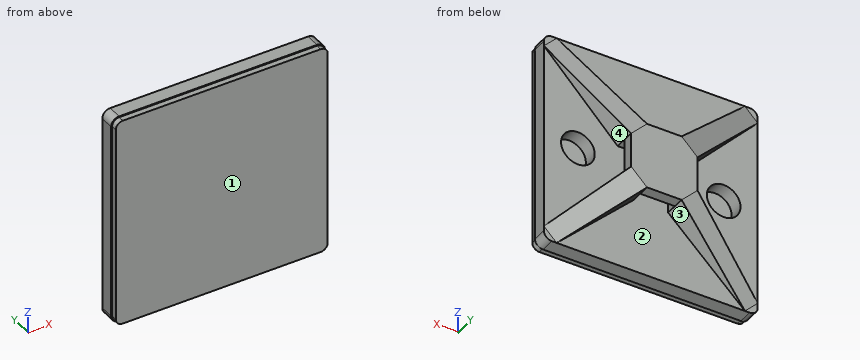
from build123d import *

# Parameters (mm, degrees)
BOSS_EXTRUDE1_DEPTH   = 1.905
BOSS_EXTRUDE2_DEPTH   = 2.921
CUT_EXTRUDE2_DEPTH    = 21.205576272
CIRPATTERN3_COUNT     = 4
SKETCH5_W             = 4.62591911
SKETCH5_H             = 1.4605
CUT_EXTRUDE3_DEPTH    = 19.7198
CIRPATTERN4_COUNT     = 4
F_8_CLEARANCE_HOLE1_D = 4.4958
BOSS_EXTRUDE3_DEPTH   = 0.79375


with BuildPart() as part:
    # Sketch1 → Boss-Extrude1 (new body)
    with BuildSketch(Plane(origin=(0, 0, 0), x_dir=(1, 0, 0), z_dir=(0, 1, 0))):
        with BuildLine():
            Line((13.2207, -14.2875), (-13.2207, -14.2875))
            ThreePointArc((-13.2207, -14.2875), (-13.975041514, -13.975041514), (-14.2875, -13.2207))
            Line((-14.2875, -13.2207), (-14.2875, 13.2207))
            ThreePointArc((-14.2875, 13.2207), (-13.975041514, 13.975041514), (-13.2207, 14.2875))
            Line((-13.2207, 14.2875), (13.2207, 14.2875))
            ThreePointArc((13.2207, 14.2875), (13.975041514, 13.975041514), (14.2875, 13.2207))
            Line((14.2875, 13.2207), (14.2875, -13.2207))
            ThreePointArc((14.2875, -13.2207), (13.975041514, -13.975041514), (13.2207, -14.2875))
        make_face()
    extrude(amount=BOSS_EXTRUDE1_DEPTH)

    # Sketch2 → Boss-Extrude2 (add)
    with BuildSketch(Plane(origin=(0, 1.905, 0), x_dir=(1, 0, 0), z_dir=(0, 1, 0))):
        Polygon((4.4323, -2.312959555), (4.4323, 2.312959555), (14.2875, 12.581251337), (12.581251337, 14.2875), (2.312959555, 4.4323), (-2.312959555, 4.4323), (-12.581251337, 14.2875), (-14.2875, 12.581251337), (-4.4323, 2.312959555), (-4.4323, -2.312959555), (-14.2875, -12.581251337), (-12.581251337, -14.2875), (-2.312959555, -4.4323), (2.312959555, -4.4323), (12.581251337, -14.2875), (14.2875, -12.581251337), align=None)
    extrude(amount=BOSS_EXTRUDE2_DEPTH)

    # Sketch4 → Cut-Extrude2 (cut, symmetric)
    with BuildSketch(Plane(origin=(0, 0, 0), x_dir=(0, -1, 0), z_dir=(0.707106781, 0, 0.707106781))):
        Polygon((-4.826, 4.769618773), (-1.905, 18.999076272), (-4.826, 18.999076272), align=None)
    cut_extrude2 = extrude(amount=CUT_EXTRUDE2_DEPTH, both=True, mode=Mode.SUBTRACT)

    # CirPattern3: Cut-Extrude2 ×4 about axis
    cirpattern3_axis = Axis((0, 0, 0), (0, 1, 0))
    for i in range(1, CIRPATTERN3_COUNT):
        add(cut_extrude2.rotate(cirpattern3_axis, i * 360 / CIRPATTERN3_COUNT), mode=Mode.SUBTRACT)

    # Sketch5 → Cut-Extrude3 (cut, through all)
    with BuildSketch(Plane.XY.offset(4.4323)):
        with Locations((0, 2.63525)):
            Rectangle(SKETCH5_W, SKETCH5_H)
    cut_extrude3 = extrude(amount=-CUT_EXTRUDE3_DEPTH, mode=Mode.SUBTRACT)

    # CirPattern4: Cut-Extrude3 ×4 about axis
    cirpattern4_axis = Axis((0, 5.0673, 0), (0, -1, 0))
    for i in range(1, CIRPATTERN4_COUNT):
        add(cut_extrude3.rotate(cirpattern4_axis, i * 360 / CIRPATTERN4_COUNT), mode=Mode.SUBTRACT)

    # 8 Clearance Hole1 (through all)
    with Locations(Plane(origin=(0, 1.905, 0), x_dir=(1, 0, 0), z_dir=(0, 1, 0))):
        with Locations((-9.7409, 0), (9.7409, 0)):
            Hole(F_8_CLEARANCE_HOLE1_D / 2)

    # Sketch6 → Boss-Extrude3 (add)
    with BuildSketch(Plane.XZ):
        with BuildLine():
            Line((-14.1605, 13.2207), (-14.1605, -13.2207))
            ThreePointArc((-14.1605, -13.2207), (-13.885238953, -13.885238953), (-13.2207, -14.1605))
            Line((-13.2207, -14.1605), (13.2207, -14.1605))
            ThreePointArc((13.2207, -14.1605), (13.885238953, -13.885238953), (14.1605, -13.2207))
            Line((14.1605, -13.2207), (14.1605, 13.2207))
            ThreePointArc((14.1605, 13.2207), (13.885238953, 13.885238953), (13.2207, 14.1605))
            Line((13.2207, 14.1605), (-13.2207, 14.1605))
            ThreePointArc((-13.2207, 14.1605), (-13.885238953, 13.885238953), (-14.1605, 13.2207))
        make_face()
    extrude(amount=BOSS_EXTRUDE3_DEPTH)


solid = part.part
Verification items for the finished model (mm, model axes). Face numbers are marked on the shaded views. Give positions to 0.01 mm unless a question says otherwise; leave off trailing zeros. Loops run counter-clockwise (first coordinate to the right, second up) from the corner with the lowest first, then second, coordinate; pieces in that order, holes last.
1) Thickness scan on line 1 along Y through (x, z) = (12.75, 3.5) (3 decimals); line 2 along X through (y, z) = (3.6, -5); line 3 along Z through (x, y) = (8, -0.25). Record the ranges inside material, lowest first.
2) Sectioned sample at C-C, the plane y = 0.7. Enter the section's corners in (x, z).
3) Depth check by flat-ended pin: pin 1 Ø0.9 at (x, y) = (5, -0.5) entering from +Z; pin 2 Ø1.6 at (x, y) = (-0.5, 4) entering from -Z; pin 3 Ø1.4 at (x, z) = (-13.5, 14) entering from +Y. Enter the tip coordinate at first touch or a pass-through.
4) Sectioned sample at B-B, the plane y = 2.25. Enter the section's corners in (x, z).
5) Draft check along Z on the marked faces 1, 2, 3 and 4. Enter one of: pulls with the +Z half, pulls with the -Z half, needs draft (parallel to the pull), parting line crosses it, or undercut.
Answers:
1. line 1: y = -0.794 to 1.905
1. line 2: x = -7.01 to -2.9, 2.9 to 7.01
1. line 3: z = -14.16 to 14.16
2. outline: (-14.29, -13.22) arc R1.07 ccw to (-13.22, -14.29) - (13.22, -14.29) arc R1.07 ccw to (14.29, -13.22) - (14.29, 13.22) arc R1.07 ccw to (13.22, 14.29) - (-13.22, 14.29) arc R1.07 ccw to (-14.29, 13.22) - close; hole circle Ø4.5 at (-9.74, 0); hole circle Ø4.5 at (9.74, 0)
3. pin 1: stops at z = 14.16
3. pin 2: stops at z = -4.43
3. pin 3: stops at y = 1.96
4. outline: (-13.12, -11.37) - (-11.37, -13.12) - (-2.31, -4.43) - (-2.31, -2.31) - (-4.43, -2.31) - close; (-13.12, 11.37) - (-4.43, 2.31) - (-2.31, 2.31) - (-2.31, 4.43) - (-11.37, 13.12) - close; (2.31, -4.43) - (11.37, -13.12) - (13.12, -11.37) - (4.43, -2.31) - (2.31, -2.31) - close; (2.31, 2.31) - (4.43, 2.31) - (13.12, 11.37) - (11.37, 13.12) - (2.31, 4.43) - close
5. face 1: needs draft
5. face 2: undercut
5. face 3: pulls with the -Z half
5. face 4: undercut
